from build123d import *

# Parameters (mm, degrees)
SKETCH1_W                                         = 152.4
SKETCH1_H                                         = 50.8
BOSS_EXTRUDE1_DEPTH                               = 6.604
FILLET1_R                                         = 25.4
SKETCH2_R                                         = 2.15265
SKETCH2_W                                         = 6.35
SKETCH2_H                                         = 6.604
CUT_EXTRUDE1_DEPTH                                = 7.604
CSK_FOR_8_FLAT_HEAD_SOCKET_CAP_SCREW1_D           = 4.3053
CSK_FOR_8_FLAT_HEAD_SOCKET_CAP_SCREW1_CSINK_D     = 9.1186
CSK_FOR_8_FLAT_HEAD_SOCKET_CAP_SCREW1_CSINK_ANGLE = 82


with BuildPart() as part:
    # Sketch1 → Boss-Extrude1 (new body)
    with BuildSketch(Plane(origin=(0, 0, 0), x_dir=(1, 0, 0), z_dir=(0, 1, 0))):
        Rectangle(SKETCH1_W, SKETCH1_H)
    extrude(amount=BOSS_EXTRUDE1_DEPTH)

    # Fillet1
    fillet1_edges = [part.edges().sort_by_distance(p)[0] for p in [
        (76.2, 3.302, 25.4),
        (-76.2, 3.302, 25.4),
    ]]
    fillet(fillet1_edges, radius=FILLET1_R)

    # Sketch2 → Cut-Extrude1 (cut, through all)
    with BuildSketch(Plane(origin=(0, 6.604, 0), x_dir=(1, 0, 0), z_dir=(0, 1, 0))):
        with Locations((-38.1, 10.16)):
            Circle(SKETCH2_R)
        with Locations((38.1, 10.16)):
            Circle(SKETCH2_R)
        with Locations((-28.575, 10.16)):
            Rectangle(SKETCH2_W, SKETCH2_H)
        with Locations((-47.625, 10.16)):
            Rectangle(SKETCH2_W, SKETCH2_H)
        with Locations((47.625, 10.16)):
            Rectangle(SKETCH2_W, SKETCH2_H)
        with Locations((28.575, 10.16)):
            Rectangle(SKETCH2_W, SKETCH2_H)
    extrude(amount=-CUT_EXTRUDE1_DEPTH, mode=Mode.SUBTRACT)

    # CSK for #8 Flat Head Socket Cap Screw1 (through all)
    with Locations(Plane(origin=(0, 6.604, 0), x_dir=(1, 0, 0), z_dir=(0, 1, 0))):
        with Locations((-38.1, 10.16), (38.1, 10.16)):
            CounterSinkHole(CSK_FOR_8_FLAT_HEAD_SOCKET_CAP_SCREW1_D / 2, CSK_FOR_8_FLAT_HEAD_SOCKET_CAP_SCREW1_CSINK_D / 2, counter_sink_angle=CSK_FOR_8_FLAT_HEAD_SOCKET_CAP_SCREW1_CSINK_ANGLE)


solid = part.part
The listing builds one solid part. Answer for the finished solid, in the listing's coordinates (mm). A direction names the side the tool comes from. Give positions to 0.01 mm unless a question says otherwise; leave off trailing zeros. Write each loop counter-clockwise with the first axis right and the second up, starting at its lowest first coordinate (ties: lowest second). Pieces come first, ordered by that corner, then holes. Notation, with made-up numbers: (16, -16) - (41, -16) arc R9 ccw to (41, -2) - close; hole circle Ø3 at (-16.5, 0). An arc over 180 degrees is marked (long way). Use a Markdown table: item, result.
1. Section A-A on z = -10.16 is taken. Count the separate pieces of the cut face and the enclosed holes in it, plus the area to 3 significant figures.
Values follow:
| item | result |
|---|---|
| separate pieces | 7 |
| enclosed holes | 0 |
| area | 769 mm² |
2. Section D-D on z = 21.5 is taken. Write down the section's boundary in (x, y).
Values follow:
| item | result |
|---|---|
| outline | (-64.32, 0) - (64.32, 0) - (64.32, 6.6) - (-64.32, 6.6) - close |
3. Find the intervals of material crossed by probe 1 along Z at (x, y) = (38.1, 2.7); probe 2 along Z at (x, y) = (28, 2.5); probe 3 along X at (y, z) = (6, -6.5), in increasing order. Write a range as from..to.
Values follow:
| item | result |
|---|---|
| probe 1 | z = -25.4..-12.31, -8.01..25.4 |
| probe 2 | z = -25.4..-13.46, -6.86..25.4 |
| probe 3 | x = -76.2..-39.8, -36.4..36.4, 39.8..76.2 |
4. A tool of negligible diameter and unlimited length cuts with its end or side. For faces 1 (the cylindrical face through (68.56, 3.35, 18.16)), 2 (the flat face through (-29, 3, -13.462)), from which of +Z, -Z, +X, -X, +Y, -Y can it reach the whole face along a straight path? Write none if from no direction.
Values follow:
| item | result |
|---|---|
| face 1 | +Z, +X, +Y, -Y |
| face 2 | +Y, -Y |
5. Each of these flat-tipped pins is pushed along its axis until it touches: P1, Ø5.5, axis at x = 38.1, z = -10.16, coming from the -Y side; P2, Ø2.5, axis at x = -38.1, z = -10.16, coming from the +Y side. Where does it stop, or does it pass through?
Values follow:
| item | result |
|---|---|
| P1 | stops at y = 0 |
| P2 | passes through |
6. Section B-B on x = -38.1 is taken. Write down the section's boundary in (y, z), plus the area to 3 significant figures.
Values follow:
| item | result |
|---|---|
| outline | (0, -25.4) - (6.6, -25.4) - (6.6, -14.72) - (3.84, -12.31) - (0, -12.31) - close; (0, -8.01) - (3.84, -8.01) - (6.6, -5.6) - (6.6, 25.4) - (0, 25.4) - close |
| area | 300 mm² |
7. Section C-C on y = 5.25 is taken. Write down the section's boundary in (x, z), plus the area to 3 significant figures.
Values follow:
| item | result |
|---|---|
| outline | (-76.2, -25.4) - (76.2, -25.4) - (76.2, 0) arc R25.4 ccw to (50.8, 25.4) - (-50.8, 25.4) arc R25.4 ccw to (-76.2, 0) - close; hole (-50.8, -13.46) - (-44.45, -13.46) - (-44.45, -6.86) - (-50.8, -6.86) - close; hole circle Ø6.76 at (-38.1, -10.16); hole (-31.75, -13.46) - (-25.4, -13.46) - (-25.4, -6.86) - (-31.75, -6.86) - close; hole (25.4, -13.46) - (31.75, -13.46) - (31.75, -6.86) - (25.4, -6.86) - close; hole circle Ø6.76 at (38.1, -10.16); hole (44.45, -13.46) - (50.8, -13.46) - (50.8, -6.86) - (44.45, -6.86) - close |
| area | 7,230 mm² |
8. For a pull along X with two mould halves and no side action, classify faces 3 (the flat face through (44.45, 3, -10)), 4 (the flat face through (76.2, 3, -13)), 5 (the flat face through (-1, 3, -25.4)) as released by +X, released by -X, zero draft, split by the parting line, or undercut.
Values follow:
| item | result |
|---|---|
| face 3 | undercut |
| face 4 | released by +X |
| face 5 | zero draft |
